from build123d import *

# Parameters (mm, degrees)
F0_W     = 60
F0_H     = 30
F0_W_2   = 59
F0_H_2   = 29
F1_DEPTH = 13
F2_DEPTH = 12
F3_R     = 1


with BuildPart() as f1:
    # F0 (on Top) → F1 (new body)
    with BuildSketch(Plane.XY):
        Rectangle(F0_W, F0_H)
        Rectangle(F0_W_2, F0_H_2, mode=Mode.SUBTRACT)
        Rectangle(F0_W_2, F0_H_2)
    extrude(amount=-F1_DEPTH)

    # F0 (on Top) → F2 (cut)
    with BuildSketch(Plane.XY):
        Rectangle(F0_W_2, F0_H_2)
    extrude(amount=-F2_DEPTH, mode=Mode.SUBTRACT)

    # F3
    f3_edges = [f1.edges().sort_by_distance(p)[0] for p in [
        (-30, 0, -13),
        (-30, 15, -6.5),
        (0, 15, -13),
        (30, 15, -6.5),
        (30, 0, -13),
        (0, -15, -13),
        (30, -15, -6.5),
        (-30, -15, -6.5),
    ]]
    fillet(f3_edges, radius=F3_R)


solid = f1.part
Read the model definition and answer for the solid it produces. Units are mm, in the model's axes. A direction names the side the tool comes from. Coordinates: 2 decimals unless noted, no trailing zeros. Write each loop counter-clockwise with the first axis right and the second up, starting at its lowest first coordinate (ties: lowest second). Pieces come first, ordered by that corner, then holes. Notation, with made-up numbers: (-21.75, 44.5) -> (-17.75, 44.5) arc R20 cw to (-17.75, 75.5) -> close; hole circle Ø9 at (39.5, -29.5). An arc over 180 degrees is marked (long way). Return JSON: item names as keys, results as strings.
(1) The part is cut by section C-C on z = -3.75. Give the vertices of the cut face in (x, y), then the cut area to 3 significant figures.
Answers below:
{"outline": "(-30, -14) arc R1 ccw to (-29, -15) -> (29, -15) arc R1 ccw to (30, -14) -> (30, 14) arc R1 ccw to (29, 15) -> (-29, 15) arc R1 ccw to (-30, 14) -> close; hole (-29.5, -14.5) -> (29.5, -14.5) -> (29.5, 14.5) -> (-29.5, 14.5) -> close", "area": "88.1 mm^2"}
(2) For a pull along X with two mould halves and no side action, classify faces 1 (the flat face through (0, 0, -12)), 2 (the flat face through (30, 0, -6)), 3 (the flat face through (0, 0, -13)) as pulls with the +X half, pulls with the -X half, needs draft (parallel to the pull), parting line crosses it, or undercut.
Answers below:
{"face 1": "undercut", "face 2": "pulls with the +X half", "face 3": "needs draft"}
(3) Which of the six approach directions +Z, -Z, +X, -X, +Y, -Y give full straight-line access (tool end or side, diameter ignored) to faces 4 (the flat face through (0, 15, -6)), 5 (the flat face through (-29.5, 0, -6))?
Answers below:
{"face 4": "+Z, -Z, +X, -X, +Y", "face 5": "+Z"}
(4) This flat-tipped pin is pushed along its axis until it touches: P1, Ø8, axis at x = -13, y = -3, coming from the +Z side. Where does it stop, or does it pass through?
Answers below:
{"P1": "z = -12"}
(5) The part is cut by section B-B on y = 6.5. Give the vertices of the cut face in (x, z), then the cut area to 3 significant figures.
Answers below:
{"outline": "(-30, -12) arc R1 ccw to (-29, -13) -> (29, -13) arc R1 ccw to (30, -12) -> (30, 0) -> (29.5, 0) -> (29.5, -12) -> (-29.5, -12) -> (-29.5, 0) -> (-30, 0) -> close", "area": "71.6 mm^2"}
(6) Consider line 1 along X through (y, z) = (8.25, -6.25); line 2 along Y through (x, z) = (19, -0.75); line 3 along Z through (x, y) = (15.5, -5.5). Determine where each line is inside the solid, lowest interval first. Write a range as from..to.
Answers below:
{"line 1": "-30..-29.5, 29.5..30", "line 2": "-15..-14.5, 14.5..15", "line 3": "-13..-12"}
(7) The part is cut by section A-A on x = -6.5. Give the vertices of the cut face in (y, z).
Answers below:
{"outline": "(-15, -12) arc R1 ccw to (-14, -13) -> (14, -13) arc R1 ccw to (15, -12) -> (15, 0) -> (14.5, 0) -> (14.5, -12) -> (-14.5, -12) -> (-14.5, 0) -> (-15, 0) -> close"}
